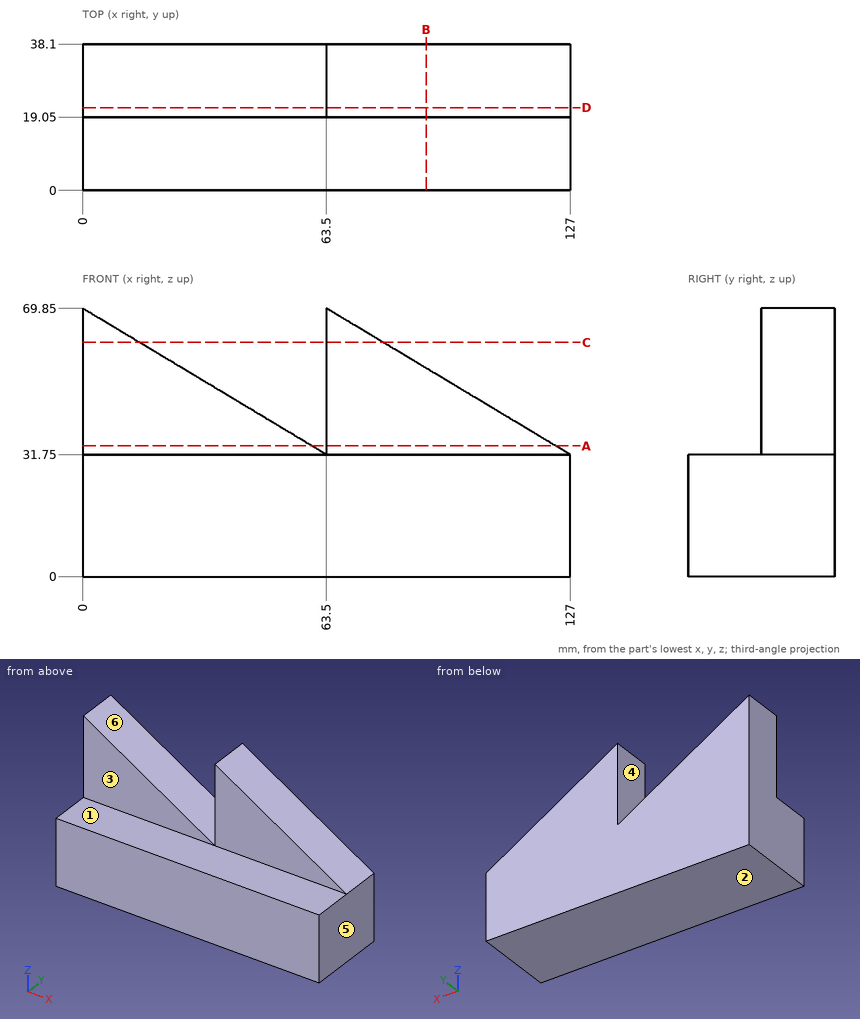
Geometry: see drawing. Coordinates: mm, zero at the bounding-box minimum. A direction names the side the tool comes from. Round coordinates to 2 decimals unless told otherwise and drop trailing zeros. Write each loop counter-clockwise with the first axis right and the second up, starting at its lowest first coordinate (ties: lowest second). Pieces come first, ordered by that corner, then holes.
Item 1: Pin query (flat end, axial travel): P1, Ø10, axis at x = 23.5, y = 26.5, coming from the +Z side; P2, Ø19, axis at x = 88.5, z = 48.5, coming from the -Y side; P3, Ø9.5, axis at x = 88, y = 8, coming from the +Z side. Return the tip coordinate at first contact, or that it passes through.
Item 2: Mould query, pull axis X, two halves, no side actions, for the marked faces 3, 4, 5 and 6. Classes: +X half, -X half, draft (parallel to the pull), parting line (faces both ways), or undercut.
Item 3: Section query B-B (x = 89.5). Return loops of the section in (y, z).
Item 4: Set-up query: the marked faces 1 and 2. Return all of +Z, -Z, +X, -X, +Y, -Y with unobstructed straight access to the full face (end or side cutting, diameter ignored); none if empty.
Item 5: Material intervals for L1, parallel to Z at x = 41, y = 17.5; L2, parallel to Y at x = 17.5, z = 33.5; L3, parallel to X at y = 21, z = 43.5, sorted ascending.
Item 6: Section query C-C (z = 61). Return loops of the section in (x, y).
Item 7: Section query D-D (y = 21.5). Return loops of the section in (x, z).
Item 8: Section query A-A (z = 34). Return loops of the section in (x, y), plus the area to 3 significant figures.
Completed:
1. P1: stops at z = 58.75
1. P2: stops at y = 19.05
1. P3: stops at z = 31.75
2. face 3: draft
2. face 4: undercut
2. face 5: +X half
2. face 6: undercut
3. outline: (0, 0) - (38.1, 0) - (38.1, 54.25) - (19.05, 54.25) - (19.05, 31.75) - (0, 31.75) - close
4. face 1: +Z, +X, -X, -Y
4. face 2: -Z, +X, -X, +Y, -Y
5. L1: z = 0 to 31.75
5. L2: y = 19.05 to 38.1
5. L3: x = 0 to 43.92, 63.5 to 107.42
6. outline: (0, 19.05) - (14.75, 19.05) - (14.75, 38.1) - (0, 38.1) - close; (63.5, 19.05) - (78.25, 19.05) - (78.25, 38.1) - (63.5, 38.1) - close
7. outline: (0, 0) - (127, 0) - (127, 31.75) - (63.5, 69.85) - (63.5, 31.75) - (0, 69.85) - close
8. outline: (0, 19.05) - (59.75, 19.05) - (59.75, 38.1) - (0, 38.1) - close; (63.5, 19.05) - (123.25, 19.05) - (123.25, 38.1) - (63.5, 38.1) - close
8. area: 2,280 mm2
